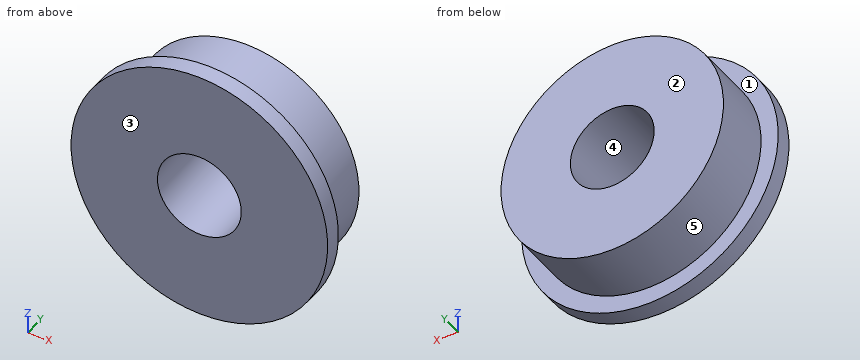
```python
from build123d import *

# Parameters (mm, degrees)
SKETCH1_R           = 7.5
BOSS_EXTRUDE1_DEPTH = 1
SKETCH2_R           = 6.5
BOSS_EXTRUDE2_DEPTH = 3.5
SKETCH3_R           = 2.45
CUT_EXTRUDE1_DEPTH  = 4.5


with BuildPart() as part:
    # Sketch1 → Boss-Extrude1 (new body)
    with BuildSketch(Plane(origin=(0, 0, 0), x_dir=(1, 0, 0), z_dir=(0, 1, 0))):
        with Locations(Location((0, 0, 0), (0, 0, 270))):
            Circle(SKETCH1_R)
    extrude(amount=BOSS_EXTRUDE1_DEPTH)

    # Sketch2 → Boss-Extrude2 (add)
    with BuildSketch(Plane(origin=(0, 1, 0), x_dir=(1, 0, 0), z_dir=(0, 1, 0))):
        with Locations(Location((0, 0, 0), (0, 0, 270))):
            Circle(SKETCH2_R)
    extrude(amount=BOSS_EXTRUDE2_DEPTH)

    # Sketch3 → Cut-Extrude1 (cut)
    with BuildSketch(Plane(origin=(0, 4.5, 0), x_dir=(1, 0, 0), z_dir=(0, 1, 0))):
        with Locations(Location((0, 0, 0), (0, 0, 270))):
            Circle(SKETCH3_R)
    extrude(amount=-CUT_EXTRUDE1_DEPTH, mode=Mode.SUBTRACT)


solid = part.part
```
Input: part model. Units: mm. Frame: model coordinates. Face numbers are marked on the shaded views. A direction names the side the tool comes from. Coordinates: 2 decimals unless noted, no trailing zeros. Loops run counter-clockwise (first coordinate to the right, second up) from the corner with the lowest first, then second, coordinate; pieces in that order, holes last. Notation, with made-up numbers: M 56,75.25 L 100,75.25 A9 cw 100,82.25 Z; hole C 44,85.5 d10. An arc over 180 degrees is marked long. Use a Markdown table: item, result. Add a question column.
1) Section A-A, the plane z = 0. Return the cut outline in (x, y), plus the area to 4 significant figures.
2) Set-up query: the marked faces 1 and 2. Return all of +Z, -Z, +X, -X, +Y, -Y with unobstructed straight access to the full face (end or side cutting, diameter ignored); none if empty.
3) Section D-D, the plane z = -3.5. Return the cut outline in (x, y), plus the area to 3 significant figures.
4) Draft query along Z for the marked faces 3, 4 and 5. Return one class per face: +Z half, -Z half, draft (parallel to the pull), parting line (faces both ways), or undercut.
5) Section C-C, the plane y = 1.65. Return the cut outline in (x, z), plus the area to 3 significant figures.
6) Pin query (flat end, axial travel): P1, Ø4.5, axis at x = 0, z = 0, coming from the -Y side; P2, Ø2, axis at x = -2, y = 1.5, coming from the +Z side; P3, Ø1.5, axis at y = 3.5, z = 2.5, coming from the -X side; P4, Ø1, axis at x = -6, y = 2.5, coming from the +Z side. Return the tip coordinate at first contact, or that it passes through.
7) Line query: L1, parallel to X at y = 3, z = 0; L2, parallel to Z at x = -1.25, y = 0.4; L3, parallel to Z at x = 1, y = 3.85. Output: solid intervals per line, ascending. Write a range as from..to.
8) Section B-B, the plane x = 0. Return the cut outline in (y, z), plus the area to 4 significant figures.
Answer below:
| question | item | result |
|---|---|---|
| 1 | outline | M -7.5,0 L -2.45,0 L -2.45,4.5 L -6.5,4.5 L -6.5,1 L -7.5,1 Z; M 2.45,0 L 7.5,0 L 7.5,1 L 6.5,1 L 6.5,4.5 L 2.45,4.5 Z |
| 1 | area | 38.45 mm2 |
| 2 | face 1 | +Y |
| 2 | face 2 | +Z, -Z, +X, -X, +Y |
| 3 | outline | M -6.63,0 L 6.63,0 L 6.63,1 L 5.48,1 L 5.48,4.5 L -5.48,4.5 L -5.48,1 L -6.63,1 Z |
| 3 | area | 51.6 mm2 |
| 4 | face 3 | draft |
| 4 | face 4 | undercut |
| 4 | face 5 | parting line |
| 5 | outline | C 0,0 d13; hole C 0,0 d4.9 |
| 5 | area | 114 mm2 |
| 6 | P1 | through |
| 6 | P2 | z = 7.41 |
| 6 | P3 | x = -6.26 |
| 6 | P4 | z = 3.46 |
| 7 | L1 | -6.5..-2.45, 2.45..6.5 |
| 7 | L2 | -7.4..-2.11, 2.11..7.4 |
| 7 | L3 | -6.42..-2.24, 2.24..6.42 |
| 8 | outline | M 0,-7.5 L 1,-7.5 L 1,-6.5 L 4.5,-6.5 L 4.5,-2.45 L 0,-2.45 Z; M 0,2.45 L 4.5,2.45 L 4.5,6.5 L 1,6.5 L 1,7.5 L 0,7.5 Z |
| 8 | area | 38.45 mm2 |
